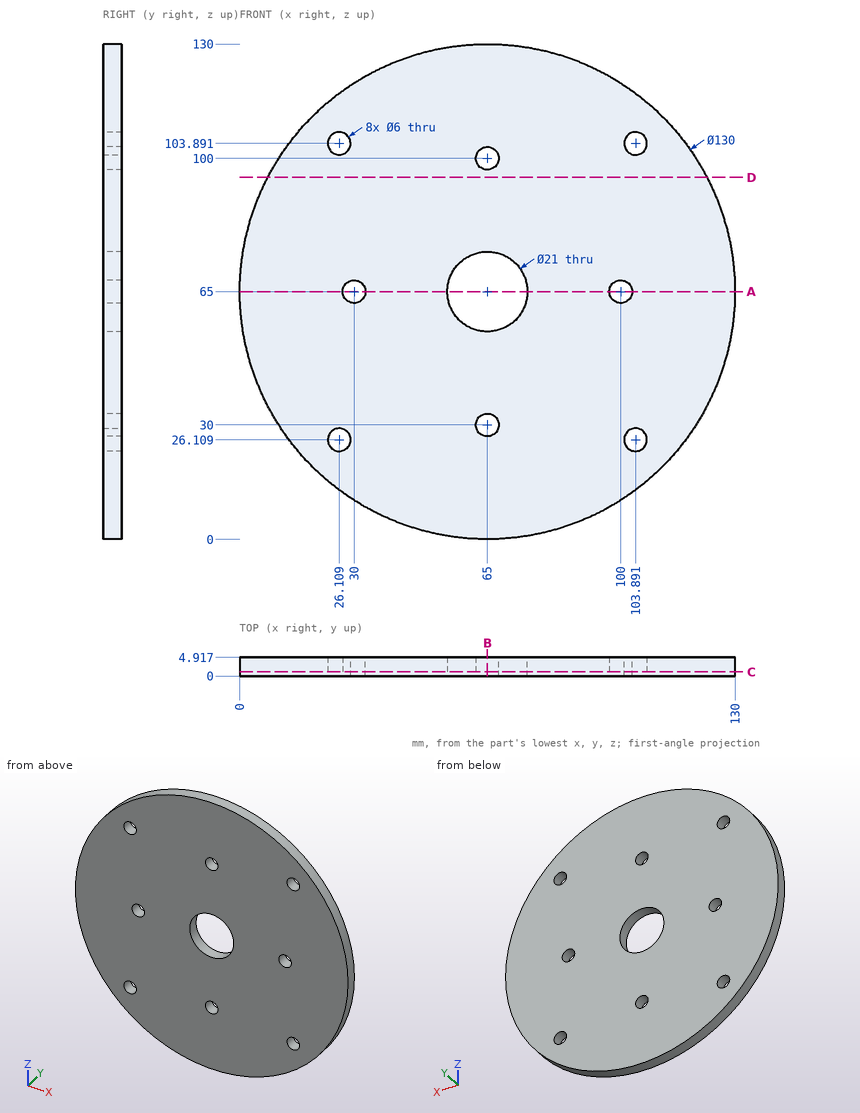
Design review of the part shown in the three views and the two pictorial views. Dimensions are in mm from the part's minimum x, y and z. Round coordinates to 2 decimals unless told otherwise and drop trailing zeros. Loops run counter-clockwise (first coordinate to the right, second up) from the corner with the lowest first, then second, coordinate; pieces in that order, holes last. Notation, with made-up numbers: (41.25, 48) - (72.25, 48) arc R15 ccw to (72.25, 59) - close; hole circle Ø1 at (49, 15). An arc over 180 degrees is marked (long way). Write each question's results on one line, items separated by ' | '. Start each with the question number.
Q1. Wall thickness on line 1 along X through (y, z) = (2.7, 65); line 2 along X through (y, z) = (3.95, 64): over which ranges is each line inside the solid? List them lowest first. Write a range as [from, to].
Q2. Take a section at C-C on y = 1.05. Give the number of separate pieces and of enclosed holes in the cut face, plus the area to 3 significant figures.
Q3. Insertion check: P1, Ø1, axis at x = 91.5, z = 102, coming from the -Y side; P2, Ø1.5, axis at x = 25.5, y = 4, coming from the -Z side; P3, Ø1.5, axis at x = 79.5, y = 1, coming from the -Z side. Each pin has a flat end and moves straight along its axis. Give the tip position at first contact, or say it passes through.
Q4. Take a section at D-D on z = 95. Give the boundary of the cut face in (x, y).
Q5. Take a section at B-B on x = 65. Give the boundary of the cut face in (y, z).
Q6. Take a section at A-A on z = 65. Give the boundary of the cut face in (x, y).
Data:
1) line 1: x = [0, 27], [33, 54.5], [75.5, 97], [103, 130] | line 2: x = [0.01, 27.17], [32.83, 54.55], [75.45, 97.17], [102.83, 129.99]
2) separate pieces: 1 | enclosed holes: 9 | area: 12,700 mm²
3) P1: stops at y = 0 | P2: stops at z = 12.81 | P3: stops at z = 1.47
4) outline: (7.34, 0) - (122.66, 0) - (122.66, 4.92) - (7.34, 4.92) - close
5) outline: (0, 0) - (4.92, 0) - (4.92, 27) - (0, 27) - close; (0, 33) - (4.92, 33) - (4.92, 54.5) - (0, 54.5) - close; (0, 75.5) - (4.92, 75.5) - (4.92, 97) - (0, 97) - close; (0, 103) - (4.92, 103) - (4.92, 130) - (0, 130) - close
6) outline: (0, 0) - (27, 0) - (27, 4.92) - (0, 4.92) - close; (33, 0) - (54.5, 0) - (54.5, 4.92) - (33, 4.92) - close; (75.5, 0) - (97, 0) - (97, 4.92) - (75.5, 4.92) - close; (103, 0) - (130, 0) - (130, 4.92) - (103, 4.92) - close
